from build123d import *

# Parameters (mm, degrees)
BOSS_EXTRUDE1_DEPTH     = 35
BOSS_EXTRUDE3_START     = 14
BOSS_EXTRUDE3_DEPTH     = 7
BOSS_EXTRUDE4_DEPTH     = 21
CUT_EXTRUDE1_DEPTH      = 203.213347551
CUT_EXTRUDE1_DEPTH_BACK = 203.213347551
BOSS_EXTRUDE5_DEPTH     = 21
CUT_EXTRUDE2_DEPTH      = 18.5
CUT_EXTRUDE3_DEPTH      = 216.030653148
CUT_EXTRUDE3_DEPTH_BACK = 216.030653148
SKETCH4_R               = 5


with BuildPart() as part:
    # Sketch1 → Boss-Extrude1 (new body)
    with BuildSketch(Plane(origin=(0, 0, 0), x_dir=(1, 0, 0), z_dir=(0, 1, 0))):
        with BuildLine():
            ThreePointArc((-160.963685795, 32.158009367), (-134.963685795, 58.158009367), (-108.963685795, 32.158009367))
            Line((-108.963685795, 32.158009367), (-103.463685795, 32.158009367))
            ThreePointArc((-103.463685795, 32.158009367), (-108.757646875, 49.636382407), (-122.860100026, 61.239845821))
            ThreePointArc((-122.860100026, 61.239845821), (-152.442058835, 58.364048287), (-166.463685795, 32.158009367))
            Line((-166.463685795, 32.158009367), (-160.963685795, 32.158009367))
        make_face()
        with BuildLine():
            Line((-103.463685795, 32.158009367), (-108.963685795, 32.158009367))
            ThreePointArc((-108.963685795, 32.158009367), (-134.963685795, 6.158009367), (-160.963685795, 32.158009367))
            Line((-160.963685795, 32.158009367), (-166.463685795, 32.158009367))
            ThreePointArc((-166.463685795, 32.158009367), (-152.442058835, 5.951970447), (-122.860100026, 3.076172913))
            ThreePointArc((-122.860100026, 3.076172913), (-108.757646875, 14.679636327), (-103.463685795, 32.158009367))
        make_face()
        with BuildLine():
            ThreePointArc((-160.963685795, 32.158009367), (-134.963685795, 58.158009367), (-108.963685795, 32.158009367))
            Line((-108.963685795, 32.158009367), (-103.463685795, 32.158009367))
            ThreePointArc((-103.463685795, 32.158009367), (-108.757646875, 49.636382407), (-122.860100026, 61.239845821))
            ThreePointArc((-122.860100026, 61.239845821), (-152.442058835, 58.364048287), (-166.463685795, 32.158009367))
            Line((-166.463685795, 32.158009367), (-160.963685795, 32.158009367))
        make_face()
        with BuildLine():
            Line((-103.463685795, 32.158009367), (-108.963685795, 32.158009367))
            ThreePointArc((-108.963685795, 32.158009367), (-134.963685795, 6.158009367), (-160.963685795, 32.158009367))
            Line((-160.963685795, 32.158009367), (-166.463685795, 32.158009367))
            ThreePointArc((-166.463685795, 32.158009367), (-152.442058835, 5.951970447), (-122.860100026, 3.076172913))
            ThreePointArc((-122.860100026, 3.076172913), (-108.757646875, 14.679636327), (-103.463685795, 32.158009367))
        make_face()
    extrude(amount=BOSS_EXTRUDE1_DEPTH)

    # Sketch1<5> → Boss-Extrude3 (add)
    with BuildSketch(Plane(origin=(0, 0, 0), x_dir=(1, 0, 0), z_dir=(0, 1, 0)).offset(BOSS_EXTRUDE3_START)):
        with BuildLine():
            ThreePointArc((-122.860100026, 61.239845821), (-86.266022188, 49.78848691), (-48.202669322, 45.158009367))
            ThreePointArc((-48.202669322, 45.158009367), (-83.19912964, 55.451565304), (-108.65874531, 81.576601162))
            ThreePointArc((-108.65874531, 81.576601162), (-118.188423055, 88.036225168), (-129.110384746, 84.395860758))
            ThreePointArc((-129.110384746, 84.395860758), (-149.219583948, 72.338856333), (-172.624945232, 70.945905698))
            ThreePointArc((-172.624945232, 70.945905698), (-184.733648255, 66.734012722), (-187.340586928, 54.181538779))
            ThreePointArc((-187.340586928, 54.181538779), (-183.88957782, 32.158009367), (-187.340586928, 10.134479955))
            ThreePointArc((-187.340586928, 10.134479955), (-184.733648255, -2.417993988), (-172.624945232, -6.629886964))
            ThreePointArc((-172.624945232, -6.629886964), (-149.219583948, -8.022837599), (-129.110384746, -20.079842023))
            ThreePointArc((-129.110384746, -20.079842023), (-118.188423055, -23.720206433), (-108.65874531, -17.260582428))
            ThreePointArc((-108.65874531, -17.260582428), (-83.19912964, 8.86445343), (-48.202669322, 19.158009367))
            ThreePointArc((-48.202669322, 19.158009367), (-86.266022188, 14.527531824), (-122.860100026, 3.076172913))
            ThreePointArc((-122.860100026, 3.076172913), (-166.463685795, 32.158009367), (-122.860100026, 61.239845821))
        make_face()
    extrude(amount=BOSS_EXTRUDE3_DEPTH)

    # Sketch1<7> → Boss-Extrude4 (add)
    with BuildSketch(Plane(origin=(0, 0, 0), x_dir=(1, 0, 0), z_dir=(0, 1, 0))):
        with BuildLine():
            Line((97.536314205, 32.158009367), (-103.463685795, 32.158009367))
            ThreePointArc((-103.463685795, 32.158009367), (-108.757646875, 14.679636327), (-122.860100026, 3.076172913))
            ThreePointArc((-122.860100026, 3.076172913), (-86.266022188, 14.527531824), (-48.202669322, 19.158009367))
            Line((-48.202669322, 19.158009367), (85.324203099, 23.158009367))
            ThreePointArc((85.324203099, 23.158009367), (95.83616648, 21.869898036), (105.481613155, 17.496573972))
            ThreePointArc((105.481613155, 17.496573972), (99.650325963, 23.820062029), (97.536314205, 32.158009367))
        make_face()
        with BuildLine():
            ThreePointArc((-122.860100026, 61.239845821), (-108.757646875, 49.636382407), (-103.463685795, 32.158009367))
            Line((-103.463685795, 32.158009367), (97.536314205, 32.158009367))
            ThreePointArc((97.536314205, 32.158009367), (99.650325963, 40.495956705), (105.481613155, 46.819444762))
            ThreePointArc((105.481613155, 46.819444762), (95.83616648, 42.446120698), (85.324203099, 41.158009367))
            Line((85.324203099, 41.158009367), (-48.202669322, 45.158009367))
            ThreePointArc((-48.202669322, 45.158009367), (-86.266022188, 49.78848691), (-122.860100026, 61.239845821))
        make_face()
    extrude(amount=BOSS_EXTRUDE4_DEPTH)

    # Sketch2 → Cut-Extrude1 (cut, two sides: drawn at the far end of the back side and taken through both)
    with BuildSketch(Plane(origin=(-0.616610621, 0, -20.583521935), x_dir=(0.9995516053170144, 0, -0.029943084480054463), z_dir=(0.02994308448005446, 0, 0.9995516053170143)).offset(-CUT_EXTRUDE1_DEPTH_BACK)):
        Polygon((-46.940258805, 23.404897351), (-46.940258805, 21), (85.979366411, 21), (85.979366411, 12.228337878), (106.836234351, 11.5), (106.836234351, 19.899284572), (106.836234351, 23.404897351), align=None)
        with BuildLine():
            Line((85.979366411, 21), (-46.940258805, 21))
            ThreePointArc((-46.940258805, 21), (-34.706035561, 17.482188037), (-22.062538217, 16.001244325))
            Line((-22.062538217, 16.001244325), (85.979366411, 12.228337878))
            Line((85.979366411, 12.228337878), (85.979366411, 21))
        make_face()
    extrude(amount=CUT_EXTRUDE1_DEPTH + CUT_EXTRUDE1_DEPTH_BACK, mode=Mode.SUBTRACT)

    # Sketch1<8> → Boss-Extrude5 (add)
    with BuildSketch(Plane(origin=(0, 0, 0), x_dir=(1, 0, 0), z_dir=(0, 1, 0))):
        with BuildLine():
            ThreePointArc((105.481613155, 46.819444762), (99.650325963, 40.495956705), (97.536314205, 32.158009367))
            Line((97.536314205, 32.158009367), (103.036314205, 32.158009367))
            ThreePointArc((103.036314205, 32.158009367), (115.036314205, 44.158009367), (127.036314205, 32.158009367))
            Line((127.036314205, 32.158009367), (132.536314205, 32.158009367))
            ThreePointArc((132.536314205, 32.158009367), (123.374261543, 47.543997609), (105.481613155, 46.819444762))
        make_face()
        with BuildLine():
            Line((103.036314205, 32.158009367), (97.536314205, 32.158009367))
            ThreePointArc((97.536314205, 32.158009367), (99.650325963, 23.820062029), (105.481613155, 17.496573972))
            ThreePointArc((105.481613155, 17.496573972), (123.374261543, 16.772021125), (132.536314205, 32.158009367))
            Line((132.536314205, 32.158009367), (127.036314205, 32.158009367))
            ThreePointArc((127.036314205, 32.158009367), (115.036314205, 20.158009367), (103.036314205, 32.158009367))
        make_face()
        with BuildLine():
            ThreePointArc((105.481613155, 46.819444762), (99.650325963, 40.495956705), (97.536314205, 32.158009367))
            Line((97.536314205, 32.158009367), (103.036314205, 32.158009367))
            ThreePointArc((103.036314205, 32.158009367), (115.036314205, 44.158009367), (127.036314205, 32.158009367))
            Line((127.036314205, 32.158009367), (132.536314205, 32.158009367))
            ThreePointArc((132.536314205, 32.158009367), (123.374261543, 47.543997609), (105.481613155, 46.819444762))
        make_face()
        with BuildLine():
            Line((103.036314205, 32.158009367), (97.536314205, 32.158009367))
            ThreePointArc((97.536314205, 32.158009367), (99.650325963, 23.820062029), (105.481613155, 17.496573972))
            ThreePointArc((105.481613155, 17.496573972), (123.374261543, 16.772021125), (132.536314205, 32.158009367))
            Line((132.536314205, 32.158009367), (127.036314205, 32.158009367))
            ThreePointArc((127.036314205, 32.158009367), (115.036314205, 20.158009367), (103.036314205, 32.158009367))
        make_face()
    extrude(amount=BOSS_EXTRUDE5_DEPTH)

    # Mirror1: part across plane


with BuildPart() as part_1:
    add(part.part)
    add(part.part.mirror(Plane.ZX))

    # Sketch3 → Cut-Extrude2 (cut)
    with BuildSketch(Plane(origin=(0, 21, 0), x_dir=(1, 0, 0), z_dir=(0, 1, 0))):
        with BuildLine():
            Line((85.036314205, 26.158009367), (-64.963685795, 26.158009367))
            ThreePointArc((-64.963685795, 26.158009367), (-70.963685795, 32.158009367), (-64.963685795, 38.158009367))
            Line((-64.963685795, 38.158009367), (85.036314205, 38.158009367))
            ThreePointArc((85.036314205, 38.158009367), (91.036314205, 32.158009367), (85.036314205, 26.158009367))
        make_face()
    cut_extrude2 = extrude(amount=-CUT_EXTRUDE2_DEPTH, mode=Mode.SUBTRACT)

    # Mirror2: Cut-Extrude2 across plane
    add(cut_extrude2.mirror(Plane.ZX), mode=Mode.SUBTRACT)

    # Sketch4 → Cut-Extrude3 (cut, two sides: drawn at the far end of the back side and taken through both)
    with BuildSketch(Plane(origin=(0, 21, 0), x_dir=(1, 0, 0), z_dir=(0, 1, 0)).offset(-CUT_EXTRUDE3_DEPTH_BACK)):
        with Locations(Location((-174.963685795, 58.158009367, 0), (0, 0, 90))):
            Circle(SKETCH4_R)
        with Locations(Location((-174.963685795, 6.158009367, 0), (0, 0, 90))):
            Circle(SKETCH4_R)
        with Locations(Location((-119.963685795, -10.841990633, 0), (0, 0, 90))):
            Circle(SKETCH4_R)
        with Locations(Location((-119.963685795, 75.158009367, 0), (0, 0, 90))):
            Circle(SKETCH4_R)
    extrude(amount=CUT_EXTRUDE3_DEPTH + CUT_EXTRUDE3_DEPTH_BACK, mode=Mode.SUBTRACT)


solid = part_1.part
Geometry check sheet. Reference: the model listing, model coordinates, mm. A direction names the side the tool comes from. Round coordinates to 2 decimals unless told otherwise and drop trailing zeros. Write each loop counter-clockwise with the first axis right and the second up, starting at its lowest first coordinate (ties: lowest second). Pieces come first, ordered by that corner, then holes.
Item 1: Section check D-D (y = -24). Record the boundary of the cut face in (x, z), plus the area to 3 significant figures.
Determined:
outline: circle Ø63 at (-134.96, -32.16); hole circle Ø52 at (-134.96, -32.16)
area: 994 mm2
Item 2: Go/stop test with flat-tipped pins: pin 1 Ø13 at (x, z) = (-174.96, -58.16) entering from +Y; pin 2 Ø20.5 at (x, y) = (-17.5, 10.5) entering from +Z; pin 3 Ø11.5 at (x, z) = (-119.96, -75.16) entering from -Y; pin 4 Ø10 at (x, z) = (-136.5, -68) entering from -Y. Record where each tip stops, or that it passes through.
Determined:
pin 1: stops at y = 21
pin 2: stops at z = -19.77
pin 3: stops at y = -21
pin 4: stops at y = -35
Item 3: Section check C-C (z = -29). Give the number of separate pieces and of enclosed holes in the cut face, plus the area to 3 significant figures.
Determined:
separate pieces: 3
enclosed holes: 0
area: 3,890 mm2
Item 4: Section check A-A (x = -135.5). Record the boundary of the cut face in (y, z).
Determined:
outline: (-35, -63.65) - (-21, -63.65) - (-21, -79.06) - (-14, -79.06) - (-14, -63.65) - (14, -63.65) - (14, -79.06) - (21, -79.06) - (21, -63.65) - (35, -63.65) - (35, -58.15) - (-35, -58.15) - close; (-35, -6.16) - (35, -6.16) - (35, -0.66) - (21, -0.66) - (21, 14.74) - (14, 14.74) - (14, -0.66) - (-14, -0.66) - (-14, 14.74) - (-21, 14.74) - (-21, -0.66) - (-35, -0.66) - close
Item 5: Section check B-B (x = 18.5). Record the boundary of the cut face in (y, z).
Determined:
outline: (-14.56, -26.16) - (-2.5, -26.16) - (-2.5, -38.16) - (-14.55, -38.16) - (-14.54, -43.16) - (14.54, -43.16) - (14.55, -38.16) - (2.5, -38.16) - (2.5, -26.16) - (14.56, -26.16) - (14.56, -21.16) - (-14.56, -21.16) - close
Item 6: Material ranges on line 1 along X through (y, z) = (-4, -29); line 2 along Z through (x, y) = (4.5, -6); line 3 along Z through (x, y) = (63, 5), recorded low to high.
Determined:
line 1: x = -166.3 to -160.77, -109.16 to -70.07, 90.14 to 103.46, 126.61 to 132.25
line 2: z = -43.58 to -38.16, -26.16 to -20.74
line 3: z = -41.83 to -38.16, -26.16 to -22.49
Item 7: Access from +Z, -Z, +X, -X, +Y, -Y to the whole of each face (thin tool, end or side, straight path). Record for faces 4 (the face through (110.9, -21, -20.7)), 5 (the face through (-8, 10, -38.158)), 6 (the face through (91.035, -7.436, -32.29)).
Determined:
face 4: +Z, -Z, +X, -Y
face 5: +Y
face 6: -Y
Item 8: Mould release check, pull along X, two halves, no side actions. Record for faces 1 (the face through (-130, -35, -58)), 2 (the face through (-118.02, -17.45, -88.01)), 3 (the face through (-82.76, -17.45, -55.19)): +X half, -X half, draft (parallel to the pull), parting line (faces both ways), or undercut.
Determined:
face 1: draft
face 2: parting line
face 3: undercut
